```python
from build123d import *

# Parameters (mm, degrees)
SKETCH1_W           = 603.25
SKETCH1_H           = 660.4
BOSS_EXTRUDE1_DEPTH = 19.05
CHAMFER1_SIZE       = 3.81
CUT_EXTRUDE2_DEPTH  = 448.629962274
SKETCH6_R           = 4.064
CUT_EXTRUDE5_DEPTH  = 448.629962274
CUT_EXTRUDE8_DEPTH  = 448.629962274
SKETCH10_W          = 603.25
SKETCH10_H          = 12.7
CUT_EXTRUDE9_DEPTH  = 1.27


with BuildPart() as part:
    # Sketch1 → Boss-Extrude1 (new body)
    with BuildSketch(Plane(origin=(0, 0, 0), x_dir=(1, 0, 0), z_dir=(0, 1, 0))):
        Rectangle(SKETCH1_W, SKETCH1_H)
    extrude(amount=BOSS_EXTRUDE1_DEPTH)

    # Chamfer1
    chamfer1_edges = [part.edges().sort_by_distance(p)[0] for p in [
        (0, 0, 330.2),
        (-301.625, 0, 0),
        (0, 0, -330.2),
        (301.625, 0, 0),
    ]]
    chamfer(chamfer1_edges, length=CHAMFER1_SIZE)

    # Sketch3 → Cut-Extrude2 (cut, through all)
    with BuildSketch(Plane(origin=(0, 19.05, 0), x_dir=(1, 0, 0), z_dir=(0, 1, 0))):
        with BuildLine():
            Line((-250.825, 162.004445849), (-161.925, 162.004445849))
            ThreePointArc((-161.925, 162.004445849), (-157.861, 157.940445849), (-161.925, 153.876445849))
            Line((-161.925, 153.876445849), (-250.825, 153.876445849))
            ThreePointArc((-250.825, 153.876445849), (-254.889, 157.940445849), (-250.825, 162.004445849))
        make_face()
        with BuildLine():
            Line((-250.825, -123.904445849), (-161.925, -123.904445849))
            ThreePointArc((-161.925, -123.904445849), (-157.861, -119.840445849), (-161.925, -115.776445849))
            Line((-161.925, -115.776445849), (-250.825, -115.776445849))
            ThreePointArc((-250.825, -115.776445849), (-254.889, -119.840445849), (-250.825, -123.904445849))
        make_face()
    extrude(amount=-CUT_EXTRUDE2_DEPTH, mode=Mode.SUBTRACT)

    # Sketch6 → Cut-Extrude5 (cut, through all)
    with BuildSketch(Plane(origin=(0, 19.05, 0), x_dir=(1, 0, 0), z_dir=(0, 1, 0))):
        with Locations(Location((-79.375, 82.55, 0), (0, 0, 270))):
            Circle(SKETCH6_R)
        with Locations(Location((-79.375, -120.65, 0), (0, 0, 270))):
            Circle(SKETCH6_R)
    extrude(amount=-CUT_EXTRUDE5_DEPTH, mode=Mode.SUBTRACT)

    # Sketch9 → Cut-Extrude8 (cut, through all)
    with BuildSketch(Plane(origin=(0, 19.05, 0), x_dir=(1, 0, 0), z_dir=(0, 1, 0))):
        with BuildLine():
            ThreePointArc((242.118601729, -139.943450479), (232.177226853, -202.293022526), (210.263074619, -261.505099002))
            ThreePointArc((210.263074619, -261.505099002), (204.8309841, -263.382486707), (202.953596395, -257.950396188))
            ThreePointArc((202.953596395, -257.950396188), (224.314710087, -200.23263079), (234.005198531, -139.456549521))
            ThreePointArc((234.005198531, -139.456549521), (238.305350609, -135.643298401), (242.118601729, -139.943450479))
        make_face()
        with BuildLine():
            ThreePointArc((242.118601729, 101.843450479), (232.177226853, 164.193022526), (210.263074619, 223.405099002))
            ThreePointArc((210.263074619, 223.405099002), (204.8309841, 225.282486707), (202.953596395, 219.850396188))
            ThreePointArc((202.953596395, 219.850396188), (224.314710087, 162.13263079), (234.005198531, 101.356549521))
            ThreePointArc((234.005198531, 101.356549521), (238.305350609, 97.543298401), (242.118601729, 101.843450479))
        make_face()
    extrude(amount=-CUT_EXTRUDE8_DEPTH, mode=Mode.SUBTRACT)

    # Sketch10 → Cut-Extrude9 (cut)
    with BuildSketch(Plane(origin=(0, 19.05, 0), x_dir=(1, 0, 0), z_dir=(0, 1, 0))):
        with Locations((0, 298.45)):
            Rectangle(SKETCH10_W, SKETCH10_H)
        with Locations((0, -260.35)):
            Rectangle(SKETCH10_W, SKETCH10_H)
    extrude(amount=-CUT_EXTRUDE9_DEPTH, mode=Mode.SUBTRACT)


solid = part.part
```
Input: part model. Units: mm. Frame: model coordinates. A direction names the side the tool comes from. Give positions to 0.01 mm unless a question says otherwise; leave off trailing zeros. Order: outer loops, then holes, each group sorted by start corner. A loop starts at its lowest first (then second) coordinate and runs counter-clockwise, first axis right, second up.
1. Line query: probe 1 along X at (y, z) = (13.75, 120.65) (3 decimals); probe 2 along Z at (x, y) = (-244.5, 5.75); probe 3 along X at (y, z) = (5.5, -82.55) (3 decimals). Output: solid intervals per line, ascending.
Computed:
probe 1: x = -301.625 to -254.808, -157.942 to -83.439, -75.311 to 301.625
probe 2: z = -330.2 to -162, -153.88 to 115.78, 123.9 to 330.2
probe 3: x = -301.625 to -83.439, -75.311 to 301.625
2. Set-up query: faces 5 (the face through (-4, 11, -330.2)), 6 (the face through (-206, 10, -153.876)). Return all of +Z, -Z, +X, -X, +Y, -Y with unobstructed straight access to the full face (end or side cutting, diameter ignored); none if empty.
Computed:
face 5: -Z, +X, -X, +Y, -Y
face 6: +Y, -Y
3. Draft query along X for faces 1 (the face through (301.625, 11, 5)), 2 (the face through (-207, 10, -162.004)), 3 (the face through (232.4, 9.66, 201.44)), 4 (the face through (-4, 0, -5)). Return one class per face: released by +X, released by -X, zero draft, split by the parting line, or undercut.
Computed:
face 1: released by +X
face 2: undercut
face 3: undercut
face 4: zero draft
4. Cut plane A-A (z = 194.5). Return loops of the section in (x, y) (3 decimals).
Computed:
outline: (-301.625, 3.81) - (-297.815, 0) - (225.759, 0) - (225.759, 19.05) - (-301.625, 19.05) - close; (234.116, 0) - (297.815, 0) - (301.625, 3.81) - (301.625, 19.05) - (234.116, 19.05) - close
5. Pin query (flat end, axial travel): pin 1 Ø4 at (x, z) = (-136.5, -297.5) entering from +Y; pin 2 Ø6 at (x, z) = (-54.5, -169.5) entering from -Y. Return the tip coordinate at first contact, or that it passes through.
Computed:
pin 1: stops at y = 17.78
pin 2: stops at y = 0
